Build history of the part. All positions in model axes, mm. Face numbers are marked on the shaded views. A direction names the side the tool comes from. Give positions to 0.01 mm unless a question says otherwise; leave off trailing zeros. Loops run counter-clockwise (first coordinate to the right, second up) from the corner with the lowest first, then second, coordinate; pieces in that order, holes last. Notation, with made-up numbers: (78, 5.25) -> (125, 5.25) arc R13 ccw to (125, 22.25) -> close; hole circle Ø6 at (-31, 1.5). An arc over 180 degrees is marked (long way). Answer as a JSON object with one key per item and string values. Group by question number.
from build123d import *

# Parameters (mm, degrees)
F3_DEPTH = 25.4
F2_W     = 6.35
F2_H     = 3.175
F1_W     = 6.35
F1_H     = 3.175
F4_DEPTH = 25.4
F6_DEPTH = 25.4


with BuildPart() as f3:
    # F0 (on Front) → F3 (new body, symmetric)
    with BuildSketch(Plane.XZ):
        Polygon((12.7, 19.05), (-12.7, 19.05), (-19.05, 12.7), (-19.05, -12.7), (-12.7, -19.05), (12.7, -19.05), (19.05, -12.7), (19.05, 12.7), align=None)
    extrude(amount=F3_DEPTH, both=True)

    # F2 (on Front) + F1 (on Front) → F4 (cut, symmetric)
    with BuildSketch(Plane.XZ):
        with Locations((15.875, -1.5875)):
            Rectangle(F2_W, F2_H)
    with BuildSketch(Plane.XZ):
        with Locations((-15.875, -1.5875)):
            Rectangle(F1_W, F1_H)
    extrude(amount=F4_DEPTH, both=True, mode=Mode.SUBTRACT)

    # F5 (on Front) → F6 (cut, symmetric)
    with BuildSketch(Plane.XZ):
        with BuildLine():
            Line((7.62, 19.05), (-7.62, 19.05))
            Line((-7.62, 19.05), (-7.62, -6.35))
            ThreePointArc((-7.62, -6.35), (0, -13.97), (7.62, -6.35))
            Line((7.62, -6.35), (7.62, 19.05))
        make_face()
    extrude(amount=F6_DEPTH, both=True, mode=Mode.SUBTRACT)


solid = f3.part
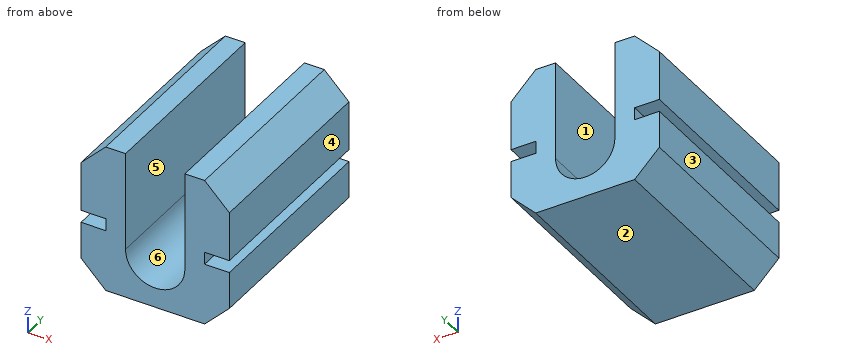
(1) Saw through at D-D on x = 0. List the corners of the cut face in (y, z).
(2) Saw through at C-C on y = -14.5. List the corners of the cut face in (x, z) (3 decimals), plus the area to 3 significant figures.
(3) Probe line 1 along X through (y, z) = (-6, 10); line 2 along X through (y, z) = (-20.5, -10); line 3 along Z through (x, y) = (14, -9) (3 decimals). List the from-to ranges inside material, lowest first. Write a range as [from, to].
(4) Pull direction X, two halves, no side cores. Call the marked faces 3, 4, 5 and 6: pulls with the +X half, pulls with the -X half, needs draft (parallel to the pull), parting line crosses it, or undercut.
(5) Pin check, flat tips, straight feed: pin 1 (1.9 mm diameter, centred on x = -15, y = 3, fed in from +Z); pin 2 (1.9 mm diameter, centred on x = 14.5, y = 5.5, fed in from +Z); pin 3 (1.9 mm diameter, centred on x = 15, y = 5.5, fed in from -Z). Stop position of each tip, or through.
(6) Saw through at B-B on z = 3. List the corners of the cut face in (x, y).
(7) Saw through at A-A on x = 14. List the corners of the cut face in (y, z) (3 decimals), plus the area to 3 significant figures.
(8) 3-axis set-ups, long thin cutter, end or side, ignore diameter. For the marked faces 1 and 2: which of +Z, -Z, +X, -X, +Y, -Y reach the whole face in a straight line?
Calculated:
{
 "1": {"outline": "(-25.4, -19.05) -> (25.4, -19.05) -> (25.4, -13.97) -> (-25.4, -13.97) -> close"},
 "2": {"outline": "(-19.05, -12.7) -> (-12.7, -19.05) -> (12.7, -19.05) -> (19.05, -12.7) -> (19.05, -3.175) -> (12.7, -3.175) -> (12.7, 0) -> (19.05, 0) -> (19.05, 12.7) -> (12.7, 19.05) -> (7.62, 19.05) -> (7.62, -6.35) arc R7.62 cw to (-7.62, -6.35) -> (-7.62, 19.05) -> (-12.7, 19.05) -> (-19.05, 12.7) -> (-19.05, 0) -> (-12.7, 0) -> (-12.7, -3.175) -> (-19.05, -3.175) -> close", "area": "852 mm^2"},
 "3": {"line 1": "x = [-19.05, -7.62], [7.62, 19.05]", "line 2": "x = [-19.05, -6.69], [6.69, 19.05]", "line 3": "z = [-17.75, -3.175], [0, 17.75]"},
 "4": {"face 3": "pulls with the -X half", "face 4": "pulls with the +X half", "face 5": "undercut", "face 6": "undercut"},
 "5": {"pin 1": "stops at z = 17.7", "pin 2": "stops at z = 18.2", "pin 3": "stops at z = -17.7"},
 "6": {"outline": "(-19.05, -25.4) -> (-7.62, -25.4) -> (-7.62, 25.4) -> (-19.05, 25.4) -> close; (7.62, -25.4) -> (19.05, -25.4) -> (19.05, 25.4) -> (7.62, 25.4) -> close"},
 "7": {"outline": "(-25.4, -17.75) -> (25.4, -17.75) -> (25.4, -3.175) -> (-25.4, -3.175) -> close; (-25.4, 0) -> (25.4, 0) -> (25.4, 17.75) -> (-25.4, 17.75) -> close", "area": "1,640 mm^2"},
 "8": {"face 1": "+Z, +Y, -Y", "face 2": "-Z, +X, -X, +Y, -Y"}
}
